from build123d import *

# Parameters (mm, degrees)
SKETCH1_R           = 14.5
SKETCH1_R_2         = 2.655602963
BOSS_EXTRUDE1_DEPTH = 10
SKETCH2_R           = 20
CUT_EXTRUDE1_DEPTH  = 2


with BuildPart() as part:
    # Sketch1 → Boss-Extrude1 (new body)
    with BuildSketch(Plane.XY):
        with BuildLine():
            Line((96.456721684, 48.36687177), (64.849048565, 79.974544889))
            Line((64.849048565, 79.974544889), (60.818539912, 84.005053542))
            ThreePointArc((60.818539912, 84.005053542), (58.909351603, 84.795865233), (57.000163293, 84.005053542))
            Line((57.000163293, 84.005053542), (25.392490174, 52.397380423))
            Line((25.392490174, 52.397380423), (21.361981522, 48.36687177))
            ThreePointArc((21.361981522, 48.36687177), (20.571169831, 46.457683461), (21.361981522, 44.548495152))
            Line((21.361981522, 44.548495152), (52.969654641, 12.940822033))
            Line((52.969654641, 12.940822033), (57.000163293, 8.91031338))
            ThreePointArc((57.000163293, 8.91031338), (58.909351603, 8.119501689), (60.818539912, 8.91031338))
            Line((60.818539912, 8.91031338), (92.426213031, 40.517986499))
            Line((92.426213031, 40.517986499), (96.456721684, 44.548495152))
            ThreePointArc((96.456721684, 44.548495152), (97.247533374, 46.457683461), (96.456721684, 48.36687177))
        make_face()
        with Locations((58.909351603, 45.077265813)):
            Circle(SKETCH1_R, mode=Mode.SUBTRACT)
        with Locations((58.909351603, 13.124669796)):
            Circle(SKETCH1_R_2, mode=Mode.SUBTRACT)
        with Locations((92.242365268, 46.457683461)):
            Circle(SKETCH1_R_2, mode=Mode.SUBTRACT)
        with Locations((58.909351603, 79.790697126)):
            Circle(SKETCH1_R_2, mode=Mode.SUBTRACT)
        with Locations((25.576337937, 46.457683461)):
            Circle(SKETCH1_R_2, mode=Mode.SUBTRACT)
    extrude(amount=BOSS_EXTRUDE1_DEPTH)

    # Sketch2 → Cut-Extrude1 (cut)
    with BuildSketch(Plane.XY.offset(10)):
        with Locations((58.909351603, 45.077265813)):
            Circle(SKETCH2_R)
    extrude(amount=-CUT_EXTRUDE1_DEPTH, mode=Mode.SUBTRACT)


solid = part.part
The model under review builds one solid part; all positions refer to its coordinate system, in mm. A direction names the side the tool comes from. Give positions to 0.01 mm unless a question says otherwise; leave off trailing zeros. Write each loop counter-clockwise with the first axis right and the second up, starting at its lowest first coordinate (ties: lowest second). Pieces come first, ordered by that corner, then holes.
1. Draft analysis for pull direction X (two halves, no side actions). For faces 1 (the flat face through (69, 56, 8)), 2 (the flat face through (73, 41, 0)), 3 (the flat face through (78.887, 65.936, 4.93)), state which applies: +X half, -X half, draft (parallel to the pull), parting line (faces both ways), or undercut.
2. Add section D-D, the plane y = 63. Write out the cut boundary in (x, z).
3. Tool access review of faces 4 (the cylindrical face through (20.57, 46.49, 4.93)), 5 (the cylindrical face through (38.93, 45.96, 9.01)): name each direction out of +Z, -Z, +X, -X, +Y, -Y from which nothing blocks a thin tool from reaching the whole face with its end or side.
4. Add section A-A, the plane x = 54.5. Write out the cut boundary in (y, z), plus the area to 3 significant figures.
5. Wall thickness on L1, parallel to X at y = 46.5, z = 1.75; L2, parallel to Y at x = 58, z = 9.25; L3, parallel to X at y = 48, z = 5: over which ranges is each line inside the solid? List them lowest first.
6. Add section B-B, the plane y = 36. Write out the cut boundary in (x, z).
7. Add section C-C, the plane z = 5.75. Write out the cut boundary in (x, y), plus the area to 3 significant figures.
8. For P1, Ø2, axis at x = 74, y = 49, coming from the +Z side; P2, Ø3, axis at x = 92.24, y = 46.46, coming from the -Z side; P3, Ø5, axis at y = 73.5, z = 2.5, coming from the -X side; P4, Ø2, axis at y = 69, z = 6, coming from the -X side, all flat-tipped, find the tip position at first contact; note any pin that passes through.
Worked answers:
1. face 1: undercut
1. face 2: draft
1. face 3: +X half
2. outline: (36, 0) - (81.82, 0) - (81.82, 10) - (67.78, 10) - (67.78, 8) - (50.03, 8) - (50.03, 10) - (36, 10) - close
3. face 4: +Z, -Z, -X
3. face 5: +Z
4. outline: (11.41, 0) - (31.26, 0) - (31.26, 8) - (25.57, 8) - (25.57, 10) - (11.41, 10) - close; (58.89, 0) - (81.5, 0) - (81.5, 10) - (64.59, 10) - (64.59, 8) - (58.89, 8) - close
4. area: 402 mm2
5. L1: x = 20.57 to 22.92, 28.23 to 44.48, 73.34 to 89.59, 94.9 to 97.25
5. L2: y = 8.28 to 10.63, 15.62 to 25.1, 65.06 to 77.3, 82.29 to 84.64
5. L3: x = 21.06 to 23.41, 27.74 to 44.71, 73.11 to 90.08, 94.4 to 96.76
6. outline: (29.91, 0) - (47.6, 0) - (47.6, 8) - (41.09, 8) - (41.09, 10) - (29.91, 10) - close; (70.22, 0) - (87.91, 0) - (87.91, 10) - (76.73, 10) - (76.73, 8) - (70.22, 8) - close
7. outline: (21.36, 44.55) - (57, 8.91) arc R2.7 ccw to (60.82, 8.91) - (96.46, 44.55) arc R2.7 ccw to (96.46, 48.37) - (60.82, 84.01) arc R2.7 ccw to (57, 84.01) - (21.36, 48.37) arc R2.7 ccw to start; hole circle Ø5.31 at (25.58, 46.46); hole circle Ø29 at (58.91, 45.08); hole circle Ø5.31 at (58.91, 13.12); hole circle Ø5.31 at (58.91, 79.79); hole circle Ø5.31 at (92.24, 46.46)
7. area: 2,360 mm2
8. P1: stops at z = 8
8. P2: passes through
8. P3: stops at x = 44
8. P4: stops at x = 41
